```python
from build123d import *

# Parameters (mm, degrees)
F0_R     = 3.0043710318
F0_R_2   = 3.175
F1_DEPTH = 25.4


with BuildPart() as f1:
    # F0 (on Top) → F1 (new body)
    with BuildSketch(Plane.XY):
        with BuildLine():
            Line((14.3825741705, 6.7199096146), (8.3514579782, 13.5006953391))
            ThreePointArc((8.3514579782, 13.5006953391), (0.3779775203, 15.8704996139), (-7.6992788751, 13.8829654542))
            Line((-7.6992788751, 13.8829654542), (-12.6724380842, 9.5616388764))
            ThreePointArc((-12.6724380842, 9.5616388764), (-15.4266258064, 3.7463103487), (-15.6463763052, -2.6844987459))
            Line((-15.6463763052, -2.6844987459), (-4.4909803426, -15.2265137363))
            ThreePointArc((-4.4909803426, -15.2265137363), (1.497725163, -15.8041907207), (7.271304677, -14.1118302603))
            ThreePointArc((7.271304677, -14.1118302603), (13.5544750313, -8.2638871983), (15.875, 0))
            ThreePointArc((15.875, 0), (15.4974028462, 3.4418207422), (14.3825741705, 6.7199096146))
        make_face()
        Circle(F0_R, mode=Mode.SUBTRACT)
        with BuildLine():
            ThreePointArc((14.3825741705, 6.7199096146), (11.861864027, 10.5504410716), (8.3514579782, 13.5006953391))
            Line((8.3514579782, 13.5006953391), (14.3825741705, 6.7199096146))
        make_face()
        with BuildLine():
            ThreePointArc((-7.6992788751, 13.8829654542), (0.3779775203, 15.8704996139), (8.3514579782, 13.5006953391))
            Line((8.3514579782, 13.5006953391), (-37.2847150373, 49.9237820037))
            ThreePointArc((-37.2847150373, 49.9237820037), (-35.9437438836, 47.1727971434), (-35.4828127154, 44.1472949049))
            ThreePointArc((-35.4828127154, 44.1472949049), (-49.345849391, 34.6861575854), (-53.1035055067, 51.0439363394))
            Line((-53.1035055067, 51.0439363394), (-86.2388696466, 31.3836151645))
            ThreePointArc((-86.2388696466, 31.3836151645), (-79.8604900877, 29.5651165544), (-77.0894247023, 23.5391842927))
            ThreePointArc((-77.0894247023, 23.5391842927), (-77.5088532877, 20.9931072211), (-78.7228126593, 18.7161066861))
            Line((-78.7228126593, 18.7161066861), (-55.225755618, 28.3622618994))
            ThreePointArc((-55.225755618, 28.3622618994), (-49.2750868032, 31.076284), (-43.3029614193, 28.4098081034))
            Line((-43.3029614193, 28.4098081034), (-20.493781308, 2.765440137))
            Line((-20.493781308, 2.765440137), (-12.6724380842, 9.5616388764))
            ThreePointArc((-12.6724380842, 9.5616388764), (-10.4125010836, 11.9831317352), (-7.6992788751, 13.8829654542))
        make_face()
        with BuildLine():
            Line((43.4916438779, -26.0074260938), (14.3825741705, 6.7199096146))
            ThreePointArc((14.3825741705, 6.7199096146), (15.4974028462, 3.4418207422), (15.875, 0))
            ThreePointArc((15.875, 0), (13.5544750313, -8.2638871983), (7.271304677, -14.1118302603))
            Line((7.271304677, -14.1118302603), (-0.7174318046, -18.2281309718))
            Line((-0.7174318046, -18.2281309718), (27.2375291318, -40.4645198026))
            ThreePointArc((27.2375291318, -40.4645198026), (26.1554745178, -32.0201927375), (31.3667877085, -25.2882007145))
            ThreePointArc((31.3667877085, -25.2882007145), (37.5361745414, -23.8446798187), (43.4916438779, -26.0074260938))
        make_face()
        with BuildLine():
            ThreePointArc((32.8070785075, -22.8069058246), (32.4209123116, -24.2414146182), (31.3667877085, -25.2882007145))
            ThreePointArc((31.3667877085, -25.2882007145), (27.4782447035, -21.3723970309), (32.8070785075, -22.8069058246))
        make_face(mode=Mode.SUBTRACT)
        with BuildLine():
            ThreePointArc((-35.4828127154, 44.1472949049), (-35.9437438836, 47.1727971434), (-37.2847150373, 49.9237820037))
            ThreePointArc((-37.2847150373, 49.9237820037), (-44.9251635555, 54.2819177239), (-53.1035055067, 51.0439363394))
            ThreePointArc((-53.1035055067, 51.0439363394), (-49.345849391, 34.6861575854), (-35.4828127154, 44.1472949049))
        make_face()
        with BuildLine():
            ThreePointArc((-15.6463763052, -2.6844987459), (-15.4266258064, 3.7463103487), (-12.6724380842, 9.5616388764))
            Line((-12.6724380842, 9.5616388764), (-20.493781308, 2.765440137))
            Line((-20.493781308, 2.765440137), (-15.6463763052, -2.6844987459))
        make_face()
        with BuildLine():
            ThreePointArc((46.5187849108, -29.4108416552), (45.1814618402, -27.5523719788), (43.4916438779, -26.0074260938))
            Line((43.4916438779, -26.0074260938), (46.5187849108, -29.4108416552))
        make_face()
        with BuildLine():
            Line((46.5187849108, -29.4108416552), (43.4916438779, -26.0074260938))
            ThreePointArc((43.4916438779, -26.0074260938), (37.5361745414, -23.8446798187), (31.3667877085, -25.2882007145))
            ThreePointArc((31.3667877085, -25.2882007145), (26.1554745178, -32.0201927375), (27.2375291318, -40.4645198026))
            ThreePointArc((27.2375291318, -40.4645198026), (39.7378929207, -45.6759099514), (47.9906570213, -34.9376807289))
            ThreePointArc((47.9906570213, -34.9376807289), (47.6163862438, -32.0779448295), (46.5187849108, -29.4108416552))
        make_face()
        with Locations((36.8781570213, -34.9376807289)):
            Circle(F0_R_2, mode=Mode.SUBTRACT)
        with BuildLine():
            ThreePointArc((-4.4909803426, -15.2265137363), (-11.861864027, -10.5504410716), (-15.6463763052, -2.6844987459))
            Line((-15.6463763052, -2.6844987459), (-20.493781308, 2.765440137))
            Line((-20.493781308, 2.765440137), (-50.4060203438, -23.2261977966))
            ThreePointArc((-50.4060203438, -23.2261977966), (-55.7132555315, -25.1967300425), (-61.0031443147, -23.1800943961))
            Line((-61.0031443147, -23.1800943961), (-80.9405468136, -10.5763001971))
            ThreePointArc((-80.9405468136, -10.5763001971), (-80.316653673, -12.4114845417), (-80.1053407242, -14.3382671104))
            ThreePointArc((-80.1053407242, -14.3382671104), (-82.2990043641, -20.1855895191), (-87.7973945716, -23.1471844681))
            Line((-87.7973945716, -23.1471844681), (-63.6023153113, -36.3445038774))
            ThreePointArc((-63.6023153113, -36.3445038774), (-55.0299997662, -32.6007067871), (-49.2884898937, -39.9855341271))
            ThreePointArc((-49.2884898937, -39.9855341271), (-49.5450658668, -41.9462448655), (-50.2975152479, -43.7749159016))
            Line((-50.2975152479, -43.7749159016), (-0.7174318046, -18.2281309718))
            Line((-0.7174318046, -18.2281309718), (-4.4909803426, -15.2265137363))
        make_face()
        with BuildLine():
            Line((-0.7174318046, -18.2281309718), (7.271304677, -14.1118302603))
            ThreePointArc((7.271304677, -14.1118302603), (1.497725163, -15.8041907207), (-4.4909803426, -15.2265137363))
            Line((-4.4909803426, -15.2265137363), (-0.7174318046, -18.2281309718))
        make_face()
        with BuildLine():
            ThreePointArc((-77.0894247023, 23.5391842927), (-79.8604900877, 29.5651165544), (-86.2388696466, 31.3836151645))
            Line((-86.2388696466, 31.3836151645), (-91.3310367453, 28.3622618994))
            ThreePointArc((-91.3310367453, 28.3622618994), (-89.8500023089, 17.2350722497), (-78.7228126593, 18.7161066861))
            ThreePointArc((-78.7228126593, 18.7161066861), (-77.5088532877, 20.9931072211), (-77.0894247023, 23.5391842927))
        make_face()
        with BuildLine():
            Line((-91.3310367453, 28.3622618994), (-86.2388696466, 31.3836151645))
            ThreePointArc((-86.2388696466, 31.3836151645), (-89.0772237094, 30.3655291567), (-91.3310367453, 28.3622618994))
        make_face()
        with BuildLine():
            ThreePointArc((-57.6597608948, -47.5684090359), (-53.4182636488, -46.759212652), (-50.2975152479, -43.7749159016))
            Line((-50.2975152479, -43.7749159016), (-57.6597608948, -47.5684090359))
        make_face()
        with BuildLine():
            Line((-57.6597608948, -47.5684090359), (-50.2975152479, -43.7749159016))
            ThreePointArc((-50.2975152479, -43.7749159016), (-49.5450658668, -41.9462448655), (-49.2884898937, -39.9855341271))
            ThreePointArc((-49.2884898937, -39.9855341271), (-55.0299997662, -32.6007067871), (-63.6023153113, -36.3445038774))
            ThreePointArc((-63.6023153113, -36.3445038774), (-63.6428329888, -43.5510667769), (-57.6597608948, -47.5684090359))
        make_face()
        with BuildLine():
            ThreePointArc((-80.1053407242, -14.3382671104), (-80.316653673, -12.4114845417), (-80.9405468136, -10.5763001971))
            ThreePointArc((-80.9405468136, -10.5763001971), (-92.7573076375, -6.2834731997), (-97.0501346349, -18.1002340237))
            Line((-97.0501346349, -18.1002340237), (-87.7973945716, -23.1471844681))
            ThreePointArc((-87.7973945716, -23.1471844681), (-82.2990043641, -20.1855895191), (-80.1053407242, -14.3382671104))
        make_face()
        with BuildLine():
            Line((-87.7973945716, -23.1471844681), (-97.0501346349, -18.1002340237))
            ThreePointArc((-97.0501346349, -18.1002340237), (-93.2523370234, -22.1427582859), (-87.7973945716, -23.1471844681))
        make_face()
    extrude(amount=F1_DEPTH)


solid = f1.part
```
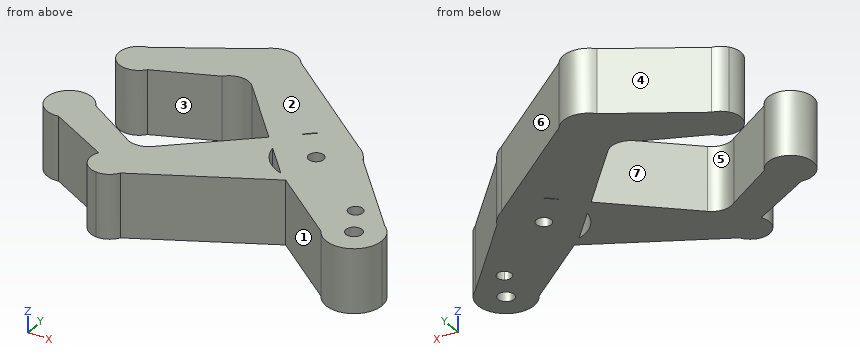
Read the model definition and answer for the solid it produces. Units are mm, in the model's axes. Face numbers are marked on the shaded views. A direction names the side the tool comes from. Give positions to 0.01 mm unless a question says otherwise; leave off trailing zeros. Write each loop counter-clockwise with the first axis right and the second up, starting at its lowest first coordinate (ties: lowest second). Pieces come first, ordered by that corner, then holes. Notation, with made-up numbers: (-15, -37) -> (40, -37) arc R21 cw to (40, -16) -> close; hole circle Ø10 at (88.5, 85). An arc over 180 degrees is marked (long way). Answer as a JSON object with one key per item and string values.
1) For a pull along X with two mould halves and no side action, classify the marked faces 4, 5, 6 and 7 as pulls with the +X half, pulls with the -X half, needs draft (parallel to the pull), parting line crosses it, or undercut.
Findings below:
{"face 4": "pulls with the -X half", "face 5": "undercut", "face 6": "pulls with the +X half", "face 7": "undercut"}
2) Straight lines are drawn through the part: probe 1 along X at (y, z) = (-11.5, 24.75); probe 2 along Y at (x, z) = (-31.5, 5); probe 3 along Y at (x, z) = (-68, 12). For each, find the intervals that lie inside material, in ascending order. Write a range as from..to.
Findings below:
{"probe 1": "x = -97.42..-79.48, -36.91..-10.94, -7.81..30.59", "probe 2": "y = -34.09..-6.8, 15.14..45.31", "probe 3": "y = -33.95..-18.76, 23.12..42.21"}
3) Section D-D on x = 10 is taken. Write down the section's boundary in (y, z), then the cut area to 3 significant figures.
Findings below:
{"outline": "(-26.75, 0) -> (12.33, 0) -> (12.33, 25.4) -> (-26.75, 25.4) -> close", "area": "993 mm^2"}
4) A tool of negligible diameter and unlimited length cuts with its end or side. For the marked faces 1, 2 and 3, from which of +Z, -Z, +X, -X, +Y, -Y can it reach the whole face along a straight path? Write none if from no direction.
Findings below:
{"face 1": "+Z, -Z, -Y", "face 2": "+Z, +X, -X, +Y, -Y", "face 3": "+Z, -Z"}
5) Section A-A on y = 0 is taken. Write down the section's boundary in (x, z).
Findings below:
{"outline": "(-23.68, 0) -> (-3, 0) -> (-3, 25.4) -> (-23.68, 25.4) -> close; (3, 0) -> (20.36, 0) -> (20.36, 25.4) -> (3, 25.4) -> close"}
6) Section B-B on z = 8.5 is taken. Count the separate pieces of the cut face and the enclosed holes in it, then the cut area to 3 significant figures.
Findings below:
{"separate pieces": "1", "enclosed holes": "5", "area": "5,690 mm^2"}
7) Section C-C on x = -70.5 is taken. Write down the section's boundary in (y, z).
Findings below:
{"outline": "(-32.58, 0) -> (-17.18, 0) -> (-17.18, 25.4) -> (-32.58, 25.4) -> close; (22.09, 0) -> (40.72, 0) -> (40.72, 25.4) -> (22.09, 25.4) -> close"}
8) Flat-ended cylindrical pins translate along their axes: pin 1 Ø6 at (x, z) = (-76.5, 10.5) entering from -Y; pin 2 Ø4 at (y, z) = (-34, 10) entering from -X; pin 3 Ø5.5 at (x, y) = (36.88, -34.94) entering from -Z; pin 4 Ø1.5 at (y, z) = (31.5, 22) entering from -X. Find the tip coordinate at first contact, or state that the pin passes through.
Findings below:
{"pin 1": "stops at y = -30.95", "pin 2": "stops at x = -71.57", "pin 3": "passes through", "pin 4": "stops at x = -88.34"}
